The listing builds one solid part. Answer for the finished solid, in the listing's coordinates (mm). A direction names the side the tool comes from. Round coordinates to 2 decimals unless told otherwise and drop trailing zeros. Order: outer loops, then holes, each group sorted by start corner. A loop starts at its lowest first (then second) coordinate and runs counter-clockwise, first axis right, second up. Notation, with made-up numbers: (21.25, 6.5) - (72.25, 6.5) arc R13 cw to (72.25, 27.5) - close; hole circle Ø3 at (17, 40). An arc over 180 degrees is marked (long way). Write item = value, one per line.
from build123d import *

# Parameters (mm, degrees)
EXTRUDE_THIN1_DEPTH = 19.05
SKETCH4_R           = 3.175
EXTRUDE3_DEPTH      = 26.527
SKETCH9_R           = 3.175
CUT_EXTRUDE3_DEPTH  = 23.352
SKETCH8_R           = 4.7625
CUT_EXTRUDE2_DEPTH  = 4.302


with BuildPart() as part:
    # Sketch1 → Extrude-Thin1 (new body, symmetric)
    with BuildSketch(Plane(origin=(0, 0, 0), x_dir=(1, 0, 0), z_dir=(0, 1, 0))):
        with BuildLine():
            Line((-19.05, -22.225), (-2.032, -22.225))
            ThreePointArc((-2.032, -22.225), (-0.595159021, -21.629840979), (0, -20.193))
            Line((0, -20.193), (0, -5.334))
            ThreePointArc((0, -5.334), (1.562292429, -1.562292429), (5.334, 0))
            Line((5.334, 0), (31.75, 0))
            Line((31.75, 0), (31.75, -3.302))
            Line((31.75, -3.302), (5.334, -3.302))
            ThreePointArc((5.334, -3.302), (3.897159021, -3.897159021), (3.302, -5.334))
            Line((3.302, -5.334), (3.302, -20.193))
            ThreePointArc((3.302, -20.193), (1.739707571, -23.964707571), (-2.032, -25.527))
            Line((-2.032, -25.527), (-19.05, -25.527))
            Line((-19.05, -25.527), (-19.05, -22.225))
        make_face()
    extrude(amount=EXTRUDE_THIN1_DEPTH, both=True)

    # Sketch4 → Extrude3 (cut, through all)
    with BuildSketch(Plane(origin=(-22.225, 0, 25.527), x_dir=(-1, 0, 0), z_dir=(0, 0, -1))):
        with Locations((-11.3792, 10.922)):
            Circle(SKETCH4_R)
        with Locations((-11.3792, -10.922)):
            Circle(SKETCH4_R)
    extrude(amount=EXTRUDE3_DEPTH, mode=Mode.SUBTRACT)

    # Sketch9 → Cut-Extrude3 (cut, through all)
    with BuildSketch(Plane(origin=(3.302, 0, 0), x_dir=(0, 0, -1), z_dir=(1, 0, 0))):
        with Locations((-12.7, 10.922)):
            Circle(SKETCH9_R)
        with Locations((-12.7, -10.922)):
            Circle(SKETCH9_R)
    extrude(amount=-CUT_EXTRUDE3_DEPTH, mode=Mode.SUBTRACT)

    # Sketch8 → Cut-Extrude2 (cut, through all)
    with BuildSketch(Plane.XY.offset(3.302)):
        with Locations((14.478, 0)):
            Circle(SKETCH8_R)
        with Locations((-55.372, 0)):
            Circle(SKETCH8_R)
    extrude(amount=-CUT_EXTRUDE2_DEPTH, mode=Mode.SUBTRACT)


solid = part.part
Q1. Section C-C on x = 18.5 is taken. Determine the outline of the cut face in (y, z).
Model answer:
outline = (-19.05, 0) - (-2.55, 0) - (-2.55, 3.3) - (-19.05, 3.3) - close; (2.55, 0) - (19.05, 0) - (19.05, 3.3) - (2.55, 3.3) - close
Q2. Determine the mould class of faces 4 (the face through (-19.05, 0, 24)), 5 (the face through (3, 19.05, 10)), 6 (the face through (1.674, -8.245, 10.993)) for opening direction Y: released by +Y, released by -Y, zero draft, split by the parting line, or undercut.
Model answer:
face_4 = zero draft
face_5 = released by +Y
face_6 = undercut
Q3. Section A-A on z = 12.7 is taken. Determine the outline of the cut face in (x, y), then the cut area to 3 significant figures.
Model answer:
outline = (0, -19.05) - (3.3, -19.05) - (3.3, -14.1) - (0, -14.1) - close; (0, -7.75) - (3.3, -7.75) - (3.3, 7.75) - (0, 7.75) - close; (0, 14.1) - (3.3, 14.1) - (3.3, 19.05) - (0, 19.05) - close
area = 83.9 mm^2
Q4. Flat-ended cylindrical pins translate along their axes: P1, Ø10, axis at y = -10.922, z = 12.7, coming from the -X side; P2, Ø21, axis at x = 20, y = 5, coming from the +Z side; P3, Ø4, axis at x = -3.5, z = 4, coming from the -Y side; P4, Ø3, axis at y = -14.5, z = 2.5, coming from the -X side. Find the tip coordinate at first contact, or state that the pin passes through.
Model answer:
P1 = 0
P2 = 3.3
P3 = through
P4 = 0.17
Q5. For faces 1 (the face through (-10, 0, 25.527)), 2 (the face through (-11, 0, 22.225)), 3 (the face through (22, 0, 3.302)), determine the directions among +Z, -Z, +X, -X, +Y, -Y from which every point of the face is accessible in a straight line to the end or side of a thin tool.
Model answer:
face_1 = +Z, +X, -X, +Y, -Y
face_2 = -Z, -X, +Y, -Y
face_3 = +Z, +X, +Y, -Y
Q6. Section D-D on y = -6.5 is taken. Determine the outline of the cut face in (x, z) (3 decimals).
Model answer:
outline = (-19.05, 22.225) - (-2.032, 22.225) arc R2.032 cw to (0, 20.193) - (0, 5.334) arc R5.334 ccw to (5.334, 0) - (31.75, 0) - (31.75, 3.302) - (5.334, 3.302) arc R2.032 cw to (3.302, 5.334) - (3.302, 20.193) arc R5.334 ccw to (-2.032, 25.527) - (-19.05, 25.527) - close
Q7. Find the intervals of material crossed by line 1 (Y direction, x = 1.2, z = 12.7); line 2 (Y direction, x = -8.5, z = 23.25); line 3 (X direction, y = 4, z = 18.75), in increasing order. Write a range as from..to.
Model answer:
line_1 = -19.05..-14.1, -7.75..7.75, 14.1..19.05
line_2 = -19.05..-13.06, -8.78..8.78, 13.06..19.05
line_3 = 0..3.3
